Print and shaded views of the part. All mm, measured from the part's lowest x, y and z. A direction names the side the tool comes from. Round coordinates to 2 decimals unless told otherwise and drop trailing zeros. Loops run counter-clockwise (first coordinate to the right, second up) from the corner with the lowest first, then second, coordinate; pieces in that order, holes last. Notation, with made-up numbers: (-24.75, -9) - (-18.75, -9) arc R5 cw to (-18.75, -4) - close; hole circle Ø6 at (70.25, 89.25). An arc over 180 degrees is marked (long way). Use one line per item in the form item = value. Start each with the question number.
Q1. Saw through at B-B (x = 12.7). Give the cut face in (y, z) (1 decimal).
Q2. Drill centre lines: line 1 (Y direction, x = 15.5, z = 15) (1 decimal); line 2 (X direction, y = 13, z = 13.75) (1 decimal); line 3 (Z direction, x = 2, y = 7) (1 decimal). Where is each one in solid material? Low to high.
Q3. Saw through at C-C (z = 10.25). Give the cut face in (x, y) (1 decimal).
Q4. 3-axis set-ups, long thin cutter, end or side, ignore diameter. For the marked faces 1, 2 and 3: which of +Z, -Z, +X, -X, +Y, -Y reach the whole face in a straight line?
Q5. Mould opens along X. For the marked faces 4, 5, 6 and 7 say: released by +X, released by -X, zero draft, split by the parting line, or undercut.
Q6. Saw through at D-D (z = 2.5). Give the cut face in (x, y) (1 decimal).
Q7. Pin check, flat tips, straight feed: pin 1 (4 mm diameter, centred on x = 3.175, z = 9.525, fed in from -Y); pin 2 (4 mm diameter, centred on x = 22.225, z = 9.525, fed in from +Y) (1 decimal); pin 3 (1.5 mm diameter, centred on x = 20.5, y = 16, fed in from +Z); pin 4 (7.5 mm diameter, centred on x = 16.5, y = 18.5, fed in from -Z). Stop position of each tip, or through.
Q8. Saw through at A-A (y = 6). Give the cut face in (x, z) (1 decimal).
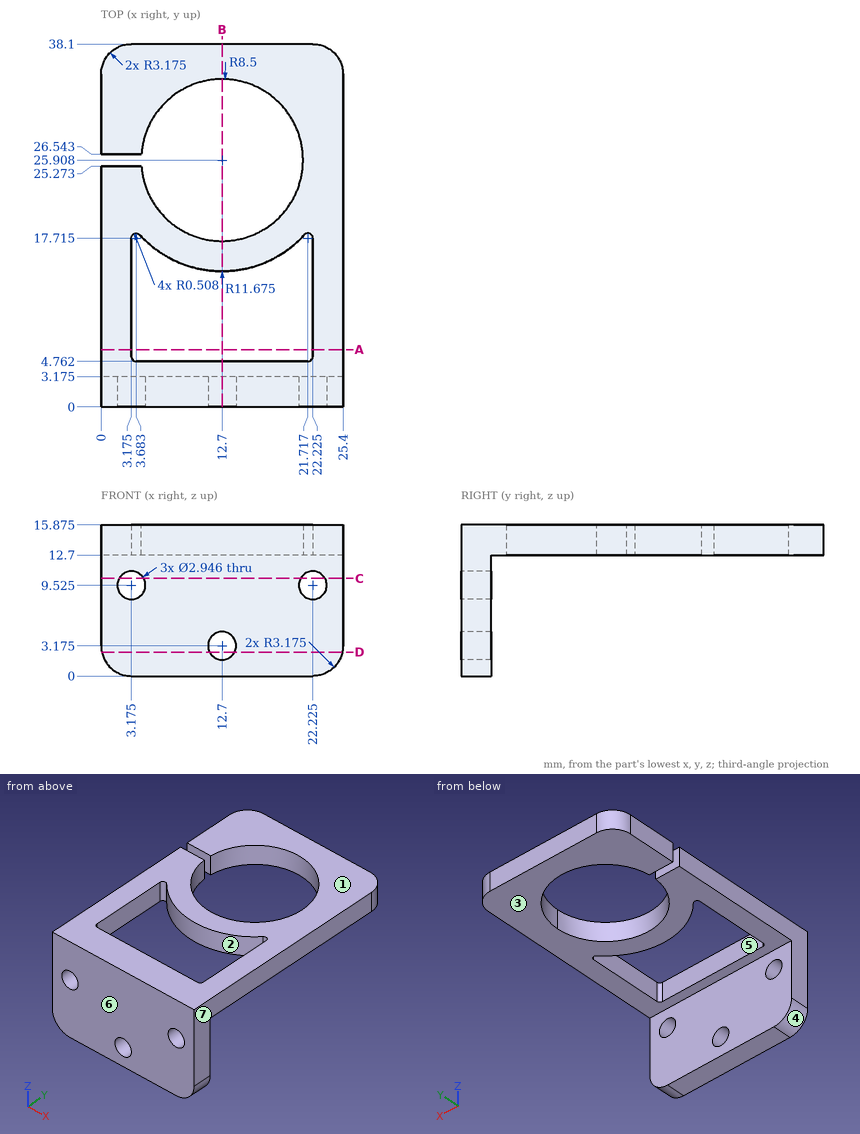
Report:
q1.outline = (0, 0) - (3.2, 0) - (3.2, 1.7) - (0, 1.7) - close; (0, 4.6) - (3.2, 4.6) - (3.2, 12.7) - (4.8, 12.7) - (4.8, 15.9) - (0, 15.9) - close; (14.2, 12.7) - (17.4, 12.7) - (17.4, 15.9) - (14.2, 15.9) - close; (34.4, 12.7) - (38.1, 12.7) - (38.1, 15.9) - (34.4, 15.9) - close
q2.line_1 = 0 to 4.8, 14.6 to 17.9, 33.9 to 38.1
q2.line_2 = 0 to 3.2, 22.2 to 25.4
q2.line_3 = 12.7 to 15.9
q3.outline = (0, 0) - (1.9, 0) - (1.9, 3.2) - (0, 3.2) - close; (4.5, 0) - (20.9, 0) - (20.9, 3.2) - (4.5, 3.2) - close; (23.5, 0) - (25.4, 0) - (25.4, 3.2) - (23.5, 3.2) - close
q4.face_1 = +Z, +X, -X, +Y, -Y
q4.face_2 = +Z, -Z
q4.face_3 = -Z, +X, -X, +Y
q5.face_4 = released by -X
q5.face_5 = undercut
q5.face_6 = zero draft
q5.face_7 = released by +X
q6.outline = (0.1, 0) - (11.4, 0) - (11.4, 3.2) - (0.1, 3.2) - close; (14, 0) - (25.3, 0) - (25.3, 3.2) - (14, 3.2) - close
q7.pin_1 = 0
q7.pin_2 = 3.2
q7.pin_3 = through
q7.pin_4 = 12.7
q8.outline = (0, 12.7) - (3.2, 12.7) - (3.2, 15.9) - (0, 15.9) - close; (22.2, 12.7) - (25.4, 12.7) - (25.4, 15.9) - (22.2, 15.9) - close
